Could you check a few things on this drawing? It's one solid part, dimensions in mm from its lowest x, y, z. Coordinates: 2 decimals unless noted, no trailing zeros. Order: outer loops, then holes, each group sorted by start corner. A loop starts at its lowest first (then second) coordinate and runs counter-clockwise, first axis right, second up.
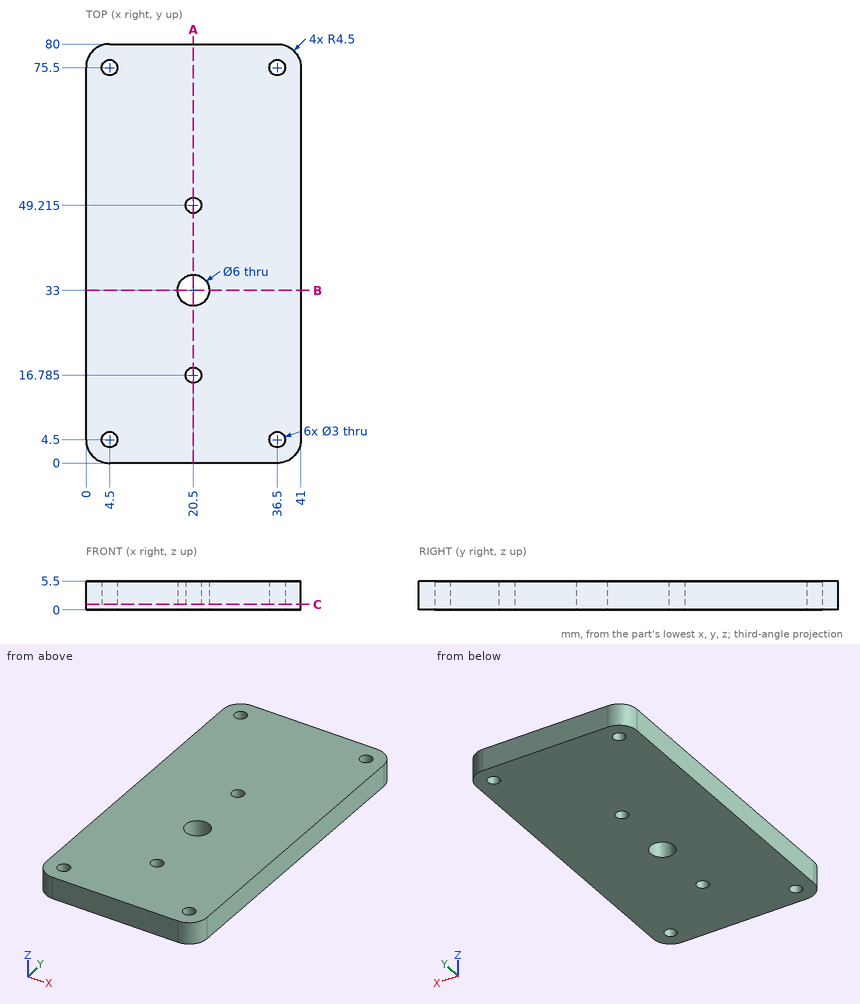
1. Imagine slicing it at B-B on y = 33. Please give me the cut outline in (x, z).
Completed:
outline: (0, 0) - (17.5, 0) - (17.5, 5.5) - (0, 5.5) - close; (23.5, 0) - (41, 0) - (41, 5.5) - (23.5, 5.5) - close
2. I'm going to push a flat-ended pin straight in: pin 1 (1.8 mm diameter, centred on x = 36.5, y = 4.5, fed in from +Z). Where does the tip first touch, or does it pass through?
Completed:
pin 1: passes through
3. Please list where these lines run through material, in increasing order: probe 1 along Y at (x, z) = (4.5, 2.55); probe 2 along Y at (x, z) = (20.5, 3.7) (3 decimals); probe 3 along X at (y, z) = (4.5, 1.6).
Completed:
probe 1: y = 0 to 3, 6 to 74, 77 to 80
probe 2: y = 0 to 15.285, 18.285 to 30, 36 to 47.715, 50.715 to 80
probe 3: x = 0 to 3, 6 to 35, 38 to 41
4. Imagine slicing it at C-C on z = 1.05. Please give me the cut outline in (x, y) (3 decimals).
Completed:
outline: (0, 4.5) arc R4.5 ccw to (4.5, 0) - (36.5, 0) arc R4.5 ccw to (41, 4.5) - (41, 75.5) arc R4.5 ccw to (36.5, 80) - (4.5, 80) arc R4.5 ccw to (0, 75.5) - close; hole circle Ø3 at (4.5, 4.5); hole circle Ø3 at (4.5, 75.5); hole circle Ø6 at (20.5, 33); hole circle Ø3 at (20.5, 16.785); hole circle Ø3 at (20.5, 49.215); hole circle Ø3 at (36.5, 4.5); hole circle Ø3 at (36.5, 75.5)
5. Imagine slicing it at A-A on x = 20.5. Please give me the cut outline in (y, z) (3 decimals).
Completed:
outline: (0, 0) - (15.285, 0) - (15.285, 5.5) - (0, 5.5) - close; (18.285, 0) - (30, 0) - (30, 5.5) - (18.285, 5.5) - close; (36, 0) - (47.715, 0) - (47.715, 5.5) - (36, 5.5) - close; (50.715, 0) - (80, 0) - (80, 5.5) - (50.715, 5.5) - close
